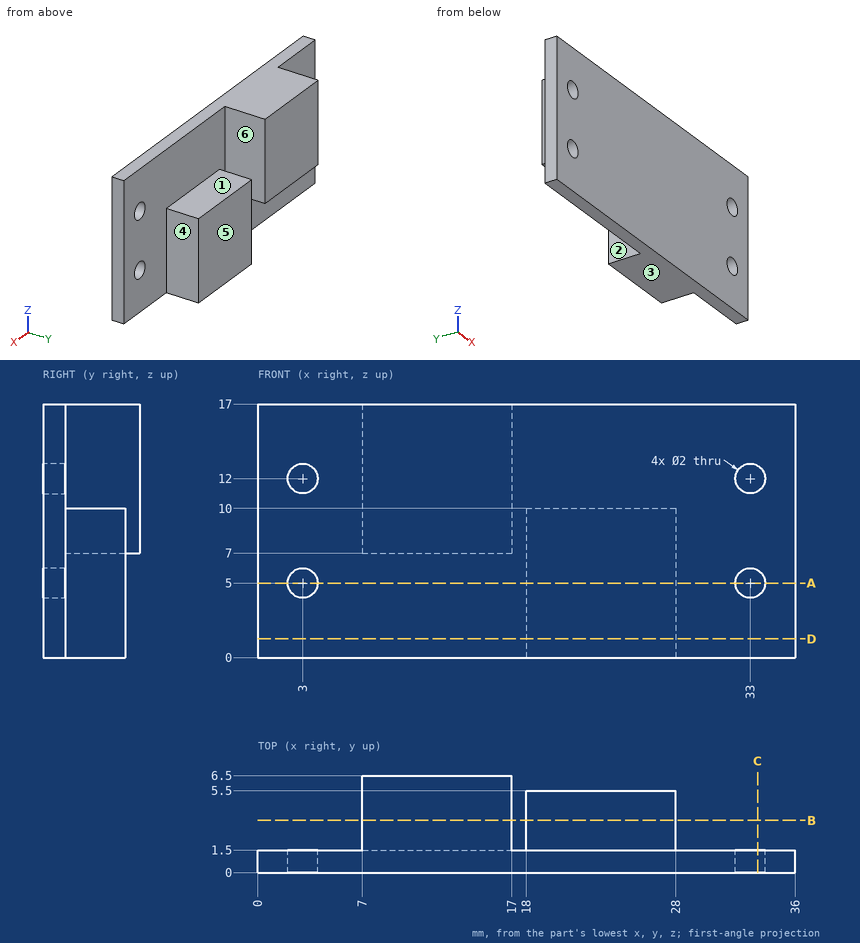
Geometry: see drawing. Coordinates: mm, zero at the bounding-box minimum. A direction names the side the tool comes from. Give positions to 0.01 mm unless a question says otherwise; leave off trailing zeros. Loops run counter-clockwise (first coordinate to the right, second up) from the corner with the lowest first, then second, coordinate; pieces in that order, holes last. Notation, with made-up numbers: (-7.5, 57.5) -> (49.5, 57.5) arc R31 ccw to (49.5, 82.5) -> close; hole circle Ø8 at (-30, 20). An arc over 180 degrees is marked (long way). Use one line per item in the form item = value.
Item 1: Draft query along X for the marked faces 4, 5 and 6. Return one class per face: pulls with the +X half, pulls with the -X half, needs draft (parallel to the pull), parting line crosses it, or undercut.
A:
face_4 = pulls with the +X half
face_5 = needs draft
face_6 = undercut
Item 2: Section query D-D on z = 1.25. Output: boundary loops of the cut face in (x, y).
A:
outline = (0, 0) -> (36, 0) -> (36, 1.5) -> (28, 1.5) -> (28, 5.5) -> (18, 5.5) -> (18, 1.5) -> (0, 1.5) -> close
Item 3: Section query A-A on z = 5. Output: boundary loops of the cut face in (x, y).
A:
outline = (0, 0) -> (2, 0) -> (2, 1.5) -> (0, 1.5) -> close; (4, 0) -> (32, 0) -> (32, 1.5) -> (28, 1.5) -> (28, 5.5) -> (18, 5.5) -> (18, 1.5) -> (4, 1.5) -> close; (34, 0) -> (36, 0) -> (36, 1.5) -> (34, 1.5) -> close
Item 4: Section query B-B on y = 3.5. Output: boundary loops of the cut face in (x, z).
A:
outline = (7, 7) -> (17, 7) -> (17, 17) -> (7, 17) -> close; (18, 0) -> (28, 0) -> (28, 10) -> (18, 10) -> close
Item 5: Pin query (flat end, axial travel): P1, Ø1.5, axis at y = 3.5, z = 11.5, coming from the -X side; P2, Ø1.5, axis at x = 11.5, y = 3.5, coming from the -Z side; P3, Ø1.2, axis at x = 21, y = 3, coming from the +Z side; P4, Ø3, axis at x = 26.5, y = 5.5, coming from the -Z side. Return the tip coordinate at first contact, or that it passes through.
A:
P1 = 7
P2 = 7
P3 = 10
P4 = 0
Item 6: Access query for the marked faces 1, 2 and 3. Directions: +Z, -Z, +X, -X, +Y, -Y. A direction counts if a zero-diameter tool reaches every point of the face in a straight line with its end or side. Return the directions, or none.
A:
face_1 = +Z, +X, +Y
face_2 = +Z, -Z, +Y
face_3 = -Z, +X, -X, +Y, -Y
Item 7: Line query: probe 1 along X at (y, z) = (0.5, 5); probe 2 along X at (y, z) = (4.25, 8.5); probe 3 along X at (y, z) = (1.25, 4.5). Output: solid intervals per line, ascending.
A:
probe_1 = 0 to 2, 4 to 32, 34 to 36
probe_2 = 7 to 17, 18 to 28
probe_3 = 0 to 2.13, 3.87 to 32.13, 33.87 to 36
Item 8: Section query C-C on x = 33.5. Output: boundary loops of the cut face in (y, z), and give its area (3 significant figures).
A:
outline = (0, 0) -> (1.5, 0) -> (1.5, 4.13) -> (0, 4.13) -> close; (0, 5.87) -> (1.5, 5.87) -> (1.5, 11.13) -> (0, 11.13) -> close; (0, 12.87) -> (1.5, 12.87) -> (1.5, 17) -> (0, 17) -> close
area = 20.3 mm^2
